```python
from build123d import *

# Parameters (mm, degrees)
SKETCH1_W           = 51.054
SKETCH1_H           = 9.525
SKETCH1_W_2         = 2.54
SKETCH1_H_2         = 3.175
BOSS_EXTRUDE1_DEPTH = 1.5
FILLET1_R           = 2.54


with BuildPart() as part:
    # Sketch1 → Boss-Extrude1 (new, symmetric)
    with BuildSketch(Plane(origin=(0, 0, 0), x_dir=(1, 0, 0), z_dir=(0, 1, 0))):
        Rectangle(SKETCH1_W, SKETCH1_H)
        with Locations((-21.082, 0)):
            Rectangle(SKETCH1_W_2, SKETCH1_H_2, mode=Mode.SUBTRACT)
        with Locations((21.082, 0)):
            Rectangle(SKETCH1_W_2, SKETCH1_H_2, mode=Mode.SUBTRACT)
    extrude(amount=BOSS_EXTRUDE1_DEPTH, both=True)

    # Fillet1
    fillet1_edges = [part.edges().sort_by_distance(p)[0] for p in [
        (-25.527, 0, -4.7625),
        (25.527, 0, -4.7625),
        (25.527, 0, 4.7625),
        (-25.527, 0, 4.7625),
    ]]
    fillet(fillet1_edges, radius=FILLET1_R)


solid = part.part
```
For this review, take the finished solid that the model builds, in its own axes (mm). A direction names the side the tool comes from. Round coordinates to 2 decimals unless told otherwise and drop trailing zeros. Write each loop counter-clockwise with the first axis right and the second up, starting at its lowest first coordinate (ties: lowest second). Pieces come first, ordered by that corner, then holes. Notation, with made-up numbers: (-26.5, -35) -> (-7.5, -35) arc R30 ccw to (-7.5, 1) -> close; hole circle Ø8 at (-5.75, 84.5). An arc over 180 degrees is marked (long way). One line per question, with ' | ' between items. Start each with the question number.
1) Machinability: for faces 4 (the flat face through (-19.812, 0, 0)), 5 (the cylindrical face through (-24.8, 0, -4)), which of the approach directions +Z, -Z, +X, -X, +Y, -Y give a long, thin tool a straight path to every point of the face, cutting with its end or side? Answer none if there is none.
2) Add section D-D (z = 3.75). Write out the cut boundary in (x, y).
3) Add section B-B (y = -0.35). Write out the cut boundary in (x, z).
4) Add section A-A (x = 21). Write out the cut boundary in (y, z), and give its area (4 significant figures).
5) Wall thickness on line 1 along X through (y, z) = (-0.65, -1.25); line 2 along X through (y, z) = (-0.1, 2.75); line 3 along X through (y, z) = (0.05, 4): over which ranges is each line inside the solid? List them lowest first.
6) Mouldability with a two-part tool opening along X and no side actions: class faces 1 (the flat face through (21, 0, 1.588)), 2 (the flat face through (0, 0, 4.762)), 3 (the cylindrical face through (-24.8, 0, 4)) as +X half, -X half, draft (parallel to the pull), parting line (faces both ways), or undercut.
7) Add section C-C (z = 0.5). Write out the cut boundary in (x, y).
Reported:
1) face 4: +Y, -Y | face 5: -Z, -X, +Y, -Y
2) outline: (-25.02, -1.5) -> (25.02, -1.5) -> (25.02, 1.5) -> (-25.02, 1.5) -> close
3) outline: (-25.53, -2.22) arc R2.54 ccw to (-22.99, -4.76) -> (22.99, -4.76) arc R2.54 ccw to (25.53, -2.22) -> (25.53, 2.22) arc R2.54 ccw to (22.99, 4.76) -> (-22.99, 4.76) arc R2.54 ccw to (-25.53, 2.22) -> close; hole (-22.35, -1.59) -> (-19.81, -1.59) -> (-19.81, 1.59) -> (-22.35, 1.59) -> close; hole (19.81, -1.59) -> (22.35, -1.59) -> (22.35, 1.59) -> (19.81, 1.59) -> close
4) outline: (-1.5, -4.76) -> (1.5, -4.76) -> (1.5, -1.59) -> (-1.5, -1.59) -> close; (-1.5, 1.59) -> (1.5, 1.59) -> (1.5, 4.76) -> (-1.5, 4.76) -> close | area: 19.05 mm²
5) line 1: x = -25.53 to -22.35, -19.81 to 19.81, 22.35 to 25.53 | line 2: x = -25.47 to 25.47 | line 3: x = -24.8 to 24.8
6) face 1: undercut | face 2: draft | face 3: -X half
7) outline: (-25.53, -1.5) -> (-22.35, -1.5) -> (-22.35, 1.5) -> (-25.53, 1.5) -> close; (-19.81, -1.5) -> (19.81, -1.5) -> (19.81, 1.5) -> (-19.81, 1.5) -> close; (22.35, -1.5) -> (25.53, -1.5) -> (25.53, 1.5) -> (22.35, 1.5) -> close
